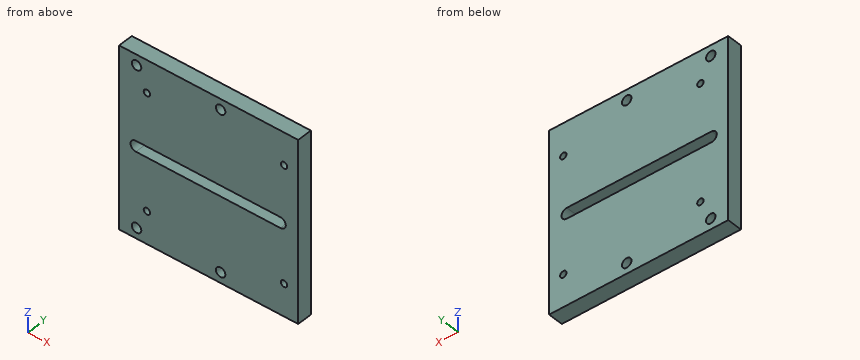
from build123d import *

# Parameters (mm, degrees)
SKETCH1_W           = 75.74480754
SKETCH1_H           = 76.2
SKETCH1_R           = 1.35
SKETCH1_R_2         = 1.999869
BOSS_EXTRUDE1_DEPTH = 6.35


with BuildPart() as part:
    # Sketch1 → Boss-Extrude1 (new body)
    with BuildSketch(Plane(origin=(0, 0, 0), x_dir=(1, 0, 0), z_dir=(0, 1, 0))):
        with Locations((-2.885014868, 0)):
            Rectangle(SKETCH1_W, SKETCH1_H)
        with Locations(Location((-29, -24.5, 0), (0, 0, 270))):
            Circle(SKETCH1_R, mode=Mode.SUBTRACT)
        with Locations(Location((29, -24.5, 0), (0, 0, 270))):
            Circle(SKETCH1_R, mode=Mode.SUBTRACT)
        with Locations(Location((-29, 24.5, 0), (0, 0, 270))):
            Circle(SKETCH1_R, mode=Mode.SUBTRACT)
        with Locations(Location((29, 24.5, 0), (0, 0, 270))):
            Circle(SKETCH1_R, mode=Mode.SUBTRACT)
        with Locations(Location((-33.386335012, 33.655, 0), (0, 0, 270))):
            Circle(SKETCH1_R_2, mode=Mode.SUBTRACT)
        with Locations(Location((-33.386335012, -33.655, 0), (0, 0, 270))):
            Circle(SKETCH1_R_2, mode=Mode.SUBTRACT)
        with Locations(Location((2.173664988, 33.655, 0), (0, 0, 270))):
            Circle(SKETCH1_R_2, mode=Mode.SUBTRACT)
        with Locations(Location((2.173664988, -33.655, 0), (0, 0, 270))):
            Circle(SKETCH1_R_2, mode=Mode.SUBTRACT)
        with BuildLine():
            Line((-33.68784786, 2.25), (27.48047437, 2.25))
            ThreePointArc((27.48047437, 2.25), (29.73047437, 0), (27.48047437, -2.25))
            Line((27.48047437, -2.25), (-33.68784786, -2.25))
            ThreePointArc((-33.68784786, -2.25), (-35.93784786, 0), (-33.68784786, 2.25))
        make_face(mode=Mode.SUBTRACT)
    extrude(amount=BOSS_EXTRUDE1_DEPTH)


solid = part.part
Part model, mm, in its own coordinate system. Coordinates: 2 decimals unless noted, no trailing zeros. Loops run counter-clockwise (first coordinate to the right, second up) from the corner with the lowest first, then second, coordinate; pieces in that order, holes last. Notation, with made-up numbers: (-28, -36) -> (-12, -36) arc R25 ccw to (-12, -1) -> close; hole circle Ø9 at (-17.5, 39.25). An arc over 180 degrees is marked (long way). Use a Markdown table: item, result. Add a question column.
Item 1: Band-saw the part on C-C on z = -24.5. Write the cut outline in (x, y).
Item 2: Band-saw the part on A-A on z = 0. Write the cut outline in (x, y).
Item 3: Band-saw the part on B-B on x = -29. Write the cut outline in (y, z).
Item 4: Band-saw the part on D-D on x = -7. Write the cut outline in (y, z).
Item 5: Flat gauge pins, fed straight in: P1, Ø3.5, axis at x = 2.17, z = 33.66, coming from the -Y side; P2, Ø4.5, axis at x = 29, z = -24.5, coming from the +Y side. Where does each tip first touch, or does it go through?
Item 6: Probe probe 1 along X at (y, z) = (2.5, -24.5); probe 2 along Z at (x, y) = (20, 6.25); probe 3 along X at (y, z) = (0.5, 0). List the from-to ranges inside material, lowest first.
Geometry says:
| question | item | result |
|---|---|---|
| 1 | outline | (-40.76, 0) -> (-30.35, 0) -> (-30.35, 6.35) -> (-40.76, 6.35) -> close; (-27.65, 0) -> (27.65, 0) -> (27.65, 6.35) -> (-27.65, 6.35) -> close; (30.35, 0) -> (34.99, 0) -> (34.99, 6.35) -> (30.35, 6.35) -> close |
| 2 | outline | (-40.76, 0) -> (-35.94, 0) -> (-35.94, 6.35) -> (-40.76, 6.35) -> close; (29.73, 0) -> (34.99, 0) -> (34.99, 6.35) -> (29.73, 6.35) -> close |
| 3 | outline | (0, -38.1) -> (6.35, -38.1) -> (6.35, -25.85) -> (0, -25.85) -> close; (0, -23.15) -> (6.35, -23.15) -> (6.35, -2.25) -> (0, -2.25) -> close; (0, 2.25) -> (6.35, 2.25) -> (6.35, 23.15) -> (0, 23.15) -> close; (0, 25.85) -> (6.35, 25.85) -> (6.35, 38.1) -> (0, 38.1) -> close |
| 4 | outline | (0, -38.1) -> (6.35, -38.1) -> (6.35, -2.25) -> (0, -2.25) -> close; (0, 2.25) -> (6.35, 2.25) -> (6.35, 38.1) -> (0, 38.1) -> close |
| 5 | P1 | through |
| 5 | P2 | y = 6.35 |
| 6 | probe 1 | -40.76 to -30.35, -27.65 to 27.65, 30.35 to 34.99 |
| 6 | probe 2 | -38.1 to -2.25, 2.25 to 38.1 |
| 6 | probe 3 | -40.76 to -35.94, 29.73 to 34.99 |
